Study the drawing (mm; zero at the part's minimum x, y, z) and answer. A direction names the side the tool comes from. Coordinates: 2 decimals unless noted, no trailing zeros. Loops run counter-clockwise (first coordinate to the right, second up) from the corner with the lowest first, then second, coordinate; pieces in that order, holes last.
Q1. The mould has two halves that part along X. Classify the marked faces 3, 4 and 5: pulls with the +X half, pulls with the -X half, needs draft (parallel to the pull), parting line crosses it, or undercut.
Q2. Flat-ended cylindrical pins translate along their axes: P1, Ø12, axis at y = 14, z = 15, coming from the -X side; P2, Ø6, axis at x = 25.5, z = 5.5, coming from the +Y side. Find the tip coordinate at first contact, or state that the pin passes through.
Q3. Section A-A (z = 5) is taken. Give the vertices of the cut face in (x, y).
Q4. Section C-C (x = 32.5) is taken. Give the vertices of the cut face in (y, z).
Q5. Section D-D (z = 18.25) is taken. Give the vertices of the cut face in (x, y), then the cut area to 3 significant figures.
Q6. Section B-B (y = 23.25) is taken. Give the vertices of the cut face in (x, z), then the cut area to 3 significant figures.
Q7. Which of the six approach directions +Z, -Z, +X, -X, +Y, -Y give full straight-line access (tool end or side, diameter ignored) to the marked faces 1 and 2?
Q8. Straight lines are drawn through the part: line 1 (Z direction, x = 32.5, y = 0.45); line 2 (X direction, y = 1.5, z = 5); line 3 (X direction, y = 6, z = 8.25). For each, find the intervals that lie inside material, in ascending order.
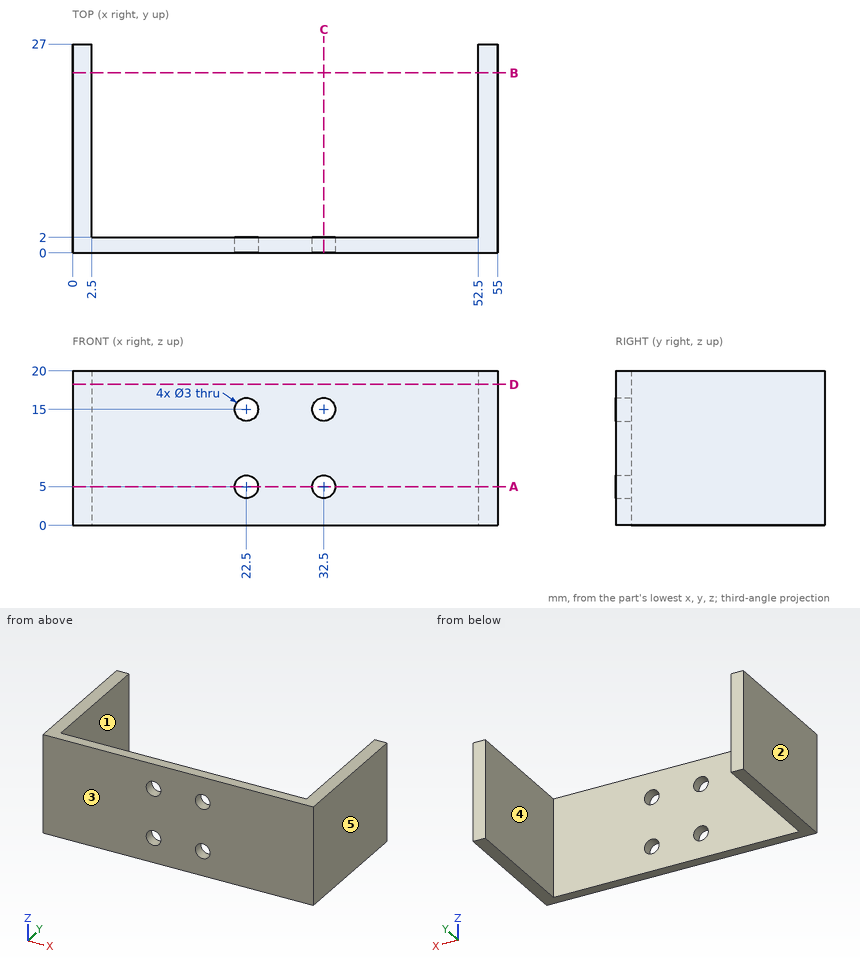
Numbers:
1. face 3: needs draft
1. face 4: undercut
1. face 5: pulls with the +X half
2. P1: stops at x = 0
2. P2: stops at y = 2
3. outline: (0, 0) - (21, 0) - (21, 2) - (2.5, 2) - (2.5, 27) - (0, 27) - close; (24, 0) - (31, 0) - (31, 2) - (24, 2) - close; (34, 0) - (55, 0) - (55, 27) - (52.5, 27) - (52.5, 2) - (34, 2) - close
4. outline: (0, 0) - (2, 0) - (2, 3.5) - (0, 3.5) - close; (0, 6.5) - (2, 6.5) - (2, 13.5) - (0, 13.5) - close; (0, 16.5) - (2, 16.5) - (2, 20) - (0, 20) - close
5. outline: (0, 0) - (55, 0) - (55, 27) - (52.5, 27) - (52.5, 2) - (2.5, 2) - (2.5, 27) - (0, 27) - close
5. area: 235 mm2
6. outline: (0, 0) - (2.5, 0) - (2.5, 20) - (0, 20) - close; (52.5, 0) - (55, 0) - (55, 20) - (52.5, 20) - close
6. area: 100 mm2
7. face 1: +Z, -Z, +Y
7. face 2: +Z, -Z, -X, +Y, -Y
8. line 1: z = 0 to 3.5, 6.5 to 13.5, 16.5 to 20
8. line 2: x = 0 to 21, 24 to 31, 34 to 55
8. line 3: x = 0 to 2.5, 52.5 to 55
